Here's how the part is built. I have some questions about the finished solid (model axes, mm). A direction names the side the tool comes from. Round coordinates to 2 decimals unless told otherwise and drop trailing zeros. Write each loop counter-clockwise with the first axis right and the second up, starting at its lowest first coordinate (ties: lowest second). Pieces come first, ordered by that corner, then holes. Notation, with made-up numbers: (47.25, 85) -> (84.25, 85) arc R14 ccw to (84.25, 93) -> close; hole circle Ø1 at (83, -1). An arc over 180 degrees is marked (long way). Put each result on its own line as item: value. Start each with the question number.
1) We'd pull the mould along X, two halves only. Please class faces 1 (the flat face through (19, 39.688, 3)), 2 (the cylindrical face through (31.68, 36.51, 3.13)), 3 (the flat face through (0, 20, 3)): released by +X, released by -X, zero draft, split by the parting line, or undercut.
2) If I drill on line 1 along X through (y, z) = (9, 1.5) (3 decimals); line 2 along Y through (x, z) = (19.05, 10); line 3 along Y through (x, z) = (19.05, 5.5), over which ranges is the centre line in solid material (lowest first)? Write a range as [from, to].
3) Will these pins go through, and if not, where does the flat tip stop? P1, Ø10, axis at x = 31.5, y = 35, coming from the +Z side; P2, Ø1, axis at y = 16, z = 19, coming from the +X side; P3, Ø9.5, axis at x = 19.05, y = 19.84, coming from the +Z side.
4) I want a section at C-C, the plane z = 3.5. Give the number of separate pieces and of enclosed holes in the cut face, then the cut area to 3 significant figures.
5) Which directions (+Z, -Z, +X, -X, +Y, -Y) give clear straight access to the entire face, cutting with the end or side of a thin tool? Please do faces 4 (the cylindrical face through (20.515, 26.174, 16.524)), 5 (the cylindrical face through (36.29, 37.78, 3.13)), 6 (the cylindrical face through (31.82, 3.176, 3.131)).
6) I want a section at B-B, the plane x = 8. List the corners of the cut face in (y, z) for me, then the cut area to 3 significant figures.
7) I want a section at A-A, the plane y = 27. List the corners of the cut face in (x, z) for me (3 decimals), then the cut area to 3 significant figures.
8) I want a section at D-D, the plane x = 26.5. List the corners of the cut face in (y, z) for me.
from build123d import *

# Parameters (mm, degrees)
BOSS_EXTRUDE1_DEPTH = 6.35
SKETCH3_R           = 6.35
BOSS_EXTRUDE2_DEPTH = 20.6375
SKETCH5_R           = 4.126342011
CUT_EXTRUDE2_DEPTH  = 62.278322577


with BuildPart() as part:
    # Sketch2 → Boss-Extrude1 (new body)
    with BuildSketch(Plane.XY):
        with BuildLine():
            Line((6.35, 0), (31.75, 0))
            ThreePointArc((31.75, 0), (36.240128061, 1.859871939), (38.1, 6.35))
            Line((38.1, 6.35), (38.1, 33.3375))
            ThreePointArc((38.1, 33.3375), (36.240128061, 37.827628061), (31.75, 39.6875))
            Line((31.75, 39.6875), (6.35, 39.6875))
            ThreePointArc((6.35, 39.6875), (1.859871939, 37.827628061), (0, 33.3375))
            Line((0, 33.3375), (0, 6.35))
            ThreePointArc((0, 6.35), (1.859871939, 1.859871939), (6.35, 0))
        make_face()
        with BuildLine():
            Line((9.525, 33.3375), (9.525, 6.35))
            ThreePointArc((9.525, 6.35), (6.35, 3.175), (3.175, 6.35))
            Line((3.175, 6.35), (3.175, 33.3375))
            ThreePointArc((3.175, 33.3375), (6.35, 36.5125), (9.525, 33.3375))
        make_face(mode=Mode.SUBTRACT)
        with BuildLine():
            Line((34.925, 33.3375), (34.925, 6.35))
            ThreePointArc((34.925, 6.35), (31.75, 3.175), (28.575, 6.35))
            Line((28.575, 6.35), (28.575, 33.3375))
            ThreePointArc((28.575, 33.3375), (31.75, 36.5125), (34.925, 33.3375))
        make_face(mode=Mode.SUBTRACT)
    extrude(amount=BOSS_EXTRUDE1_DEPTH)

    # Sketch3 → Boss-Extrude2 (add)
    with BuildSketch(Plane.XY.offset(6.35)):
        with Locations(Location((19.138936621, 19.975145899, 0), (0, 0, 180))):
            Circle(SKETCH3_R)
    extrude(amount=BOSS_EXTRUDE2_DEPTH)

    # Cut-Loft1: read off the stored shape, not the designer's step
    # Cut-Loft1: loft between two sections, ruled curve by curve
    cut_loft1_from = [
        Edge.make_bspline([(23.27505423, 15.156947986, 26.9875), (13.638658406, 6.884712768, 26.9875), (5.366423187, 16.521108592, 26.9875), (15.002819012, 24.793343811, 26.9875), (24.639214837, 33.065579029, 26.9875), (32.911450055, 23.429183205, 26.9875), (23.27505423, 15.156947986, 26.9875)], [0, 0, 0, 0, 0.5, 0.5, 0.5, 1, 1, 1, 1], 3, [1, 0.333333333, 0.333333333, 1, 0.333333333, 0.333333333, 1]),
    ]
    cut_loft1_to = [
        Edge.make_bspline([(21.665907522, 18.052896418, 22.225), (17.82140856, 12.998954616, 22.225), (12.767466759, 16.843453578, 22.225), (16.611965721, 21.89739538, 22.225), (20.456464682, 26.951337181, 22.225), (25.510406484, 23.106838219, 22.225), (21.665907522, 18.052896418, 22.225)], [0, 0, 0, 0, 0.5, 0.5, 0.5, 1, 1, 1, 1], 3, [1, 0.333333333, 0.333333333, 1, 0.333333333, 0.333333333, 1]),
    ]
    cut_loft1 = Solid(Shell([*[Face.make_surface_from_curves(cut_loft1_from[k], cut_loft1_to[k]) for k in range(1)], Face(Wire(cut_loft1_from)), Face(Wire(cut_loft1_to))]))
    add(cut_loft1, mode=Mode.SUBTRACT)

    # Sketch5 → Cut-Extrude2 (cut, through all)
    with BuildSketch(Plane(origin=(0, 0, 0), x_dir=(-1, 0, 0), z_dir=(0, 0, -1))):
        with Locations((-19.05, 19.84375)):
            Circle(SKETCH5_R)
    extrude(amount=-CUT_EXTRUDE2_DEPTH, mode=Mode.SUBTRACT)


solid = part.part
Findings:
1. face 1: zero draft
1. face 2: undercut
1. face 3: released by -X
2. line 1: x = [0, 3.175], [9.525, 28.575], [34.925, 38.1]
2. line 2: y = [13.63, 15.72], [23.97, 26.32]
2. line 3: y = [0, 15.72], [23.97, 39.69]
3. P1: stops at z = 6.35
3. P2: stops at x = 24.45
3. P3: stops at z = 24.86
4. separate pieces: 1
4. enclosed holes: 3
4. area: 1,020 mm2
5. face 4: +Z
5. face 5: +Z, -Z, +X, +Y
5. face 6: +Z, -Z
6. outline: (0, 0) -> (3.64, 0) -> (3.64, 6.35) -> (0, 6.35) -> close; (36.05, 0) -> (39.69, 0) -> (39.69, 6.35) -> (36.05, 6.35) -> close
6. area: 46.2 mm2
7. outline: (0, 0) -> (3.175, 0) -> (3.175, 6.35) -> (0, 6.35) -> close; (9.525, 0) -> (28.575, 0) -> (28.575, 6.35) -> (9.525, 6.35) -> close; (34.925, 0) -> (38.1, 0) -> (38.1, 6.35) -> (34.925, 6.35) -> close
7. area: 161 mm2
8. outline: (0, 0) -> (39.69, 0) -> (39.69, 6.35) -> (0, 6.35) -> close
